Build history of the part. All positions in model axes, mm. A direction names the side the tool comes from. Round coordinates to 2 decimals unless told otherwise and drop trailing zeros. Loops run counter-clockwise (first coordinate to the right, second up) from the corner with the lowest first, then second, coordinate; pieces in that order, holes last.
from build123d import *

# Parameters (mm, degrees)
F0_R     = 16
F1_DEPTH = 2.5
F2_R     = 16
F2_R_2   = 11.75
F3_DEPTH = 9
F4_R     = 1.5


with BuildPart() as f1:
    # F0 (on Front) → F1 (new body)
    with BuildSketch(Plane.XZ):
        Circle(F0_R)
    extrude(amount=F1_DEPTH)

    # F2 (on face) → F3 (join)
    with BuildSketch(Plane.XZ.offset(2.5)):
        Circle(F2_R)
        Circle(F2_R_2, mode=Mode.SUBTRACT)
    extrude(amount=F3_DEPTH)

    # F4
    f4_edges = [f1.edges().sort_by_distance(p)[0] for p in [
        (-16, 0, 0),
    ]]
    fillet(f4_edges, radius=F4_R)


solid = f1.part
(1) Which spindle directions (+Z, -Z, +X, -X, +Y, -Y) get a long thin tool onto all of the face, cutting with end or side? Do faces 1 (the face through (0, -2.5, 0)), 2 (the face through (0, -11.5, 12)). Say none if no direction does.
Responses:
face 1: -Y
face 2: +Z, -Z, +X, -X, -Y
(2) Slice it at C-C on y = -6.25. List the corners of the cut face in (x, z), plus the area to 3 significant figures.
Responses:
outline: circle Ø32 at (0, 0); hole circle Ø23.5 at (0, 0)
area: 371 mm2
(3) Slice it at A-A on x = 0. List the corners of the cut face in (y, z).
Responses:
outline: (-11.5, -16) - (-1.5, -16) arc R1.5 ccw to (0, -14.5) - (0, 14.5) arc R1.5 ccw to (-1.5, 16) - (-11.5, 16) - (-11.5, 11.75) - (-2.5, 11.75) - (-2.5, -11.75) - (-11.5, -11.75) - close
(4) Slice it at D-D on y = -2. List the corners of the cut face in (x, z), plus the area to 3 significant figures.
Responses:
outline: circle Ø32 at (0, 0)
area: 804 mm2
(5) Slice it at B-B on z = 0. List the corners of the cut face in (x, y), plus the area to 3 significant figures.
Responses:
outline: (-16, -11.5) - (-11.75, -11.5) - (-11.75, -2.5) - (11.75, -2.5) - (11.75, -11.5) - (16, -11.5) - (16, -1.5) arc R1.5 ccw to (14.5, 0) - (-14.5, 0) arc R1.5 ccw to (-16, -1.5) - close
area: 156 mm2
(6) Pin check, flat tips, straight feed: P1, Ø1, axis at x = -4.5, y = -3, coming from the +Z side; P2, Ø4, axis at y = -6, z = 12, coming from the +X side; P3, Ø14, axis at x = 0, z = 0, coming from the -Y side. Stop position of each tip, or through.
Responses:
P1: stops at z = 15.49
P2: stops at x = 12.49
P3: stops at y = -2.5
(7) Probe line 1 (Z direction, x = 0, y = -5.5); line 2 (Y direction, x = 1, z = -5.5); line 3 (X direction, y = -3.25, z = 3). List the from-to ranges inside material, lowest first.
Responses:
line 1: z = -16 to -11.75, 11.75 to 16
line 2: y = -2.5 to 0
line 3: x = -15.72 to -11.36, 11.36 to 15.72
(8) Pull direction Z, two halves, no side cores. Call faces 3 (the face through (0, 0, 0)), 4 (the face through (11.207, -6.937, 3.529)), 5 (the face through (-3.47, -6.43, -15.62)): +Z half, -Z half, draft (parallel to the pull), parting line (faces both ways), or undercut.
Responses:
face 3: draft
face 4: undercut
face 5: parting line
